Source: CAD feature listing. Evaluate the final solid. Frame: model axes, mm. A direction names the side the tool comes from. Give positions to 0.01 mm unless a question says otherwise; leave off trailing zeros. Order: outer loops, then holes, each group sorted by start corner. A loop starts at its lowest first (then second) coordinate and runs counter-clockwise, first axis right, second up.
1) Draft query along X for faces 1 (the face through (-33.44, 75.56, -0.99)), 2 (the face through (-60, 11, -1)), 3 (the face through (-91.38, 62.7, -0.99)), 4 (the face through (-33, 44, -2)). Return one class per face: released by +X, released by -X, zero draft, split by the parting line, or undercut.
2) Section C-C, the plane x = -45.5. Return loops of the section in (y, z).
3) Section B-B, the plane y = 78.5. Return loops of the section in (x, z).
4) Material intervals for line 1 (X direction, y = 45, z = -1); line 2 (Y direction, x = 27.5, z = 4.5); line 3 (Z direction, x = -79.5, y = 46.5), sorted ascending.
5) Access query for faces 5 (the face through (-33, 44, 0)), 6 (the face through (-60.1, 71.67, -0.99)), 7 (the face through (60, 11, -1)). Directions: +Z, -Z, +X, -X, +Y, -Y. A direction counts if a zero-diameter tool reaches every point of the face in a straight line with its end or side. Return the directions, or none.
6) Section A-A, the plane x = -81.5. Return loops of the section in (y, z), plus the area to 3 significant figures.
7) Section D-D, the plane z = 3. Return loops of the section in (x, y), plus the area to 3 significant figures.
8) First-contact query: P1, Ø5, axis at x = -102, z = -0.5, coming from the +Y side; P2, Ø2, axis at y = 31, z = -0.5, coming from the -X side; P3, Ø2, axis at y = 16.5, z = 0.5, coming from the -X side; P4, Ø1, axis at y = 62, z = 2, coming from the +X side. Flat tips, straight axial feed; report the tip coordinate or a pass-through.
Autodesk Inventor part; units mm, degrees
ref_plane "YZ Plane" through (0, 0, 0) normal (1, 0, 0) x (0, 1, 0)
ref_plane "XZ Plane" through (0, 0, 0) normal (0, 1, 0) x (-1, 0, 0)
ref_plane "XY Plane" through (0, 0, 0) normal (0, 0, 1) x (1, 0, 0)
sketch "草圖1" plane through (0, 0, 0) normal (0, 0, 1) x (1, 0, 0)
  line L0 (0, 0) -> (-40.5681, 0) construction
  line L1 (0, 0) -> (0, 45.2738) construction
  line L2 (-60, 18.7) -> (-21.9145, 18.7) construction
  line L3 (60, 18.1203) -> (60, 3.5)
  line L4 (56.5, 0) -> (-56.5, 0)
  line L5 (-60, 3.5) -> (-60, 18.7)
  line L6 (-87.6368, 8.7) -> (76.2221, 8.7)
  arc A0 (-60, 3.5) -> (-56.5, 0) centre (-56.5, 3.5) ccw
  arc A1 (56.5, 0) -> (60, 3.5) centre (56.5, 3.5) ccw
  arc A2 (-25, 17.157) -> (25, 17.157) centre (0, 60.4582) ccw
  line L7 (-27.5, 18.7) -> (27.5, 18.7) construction
  line L8 (16.8799, 18.7) -> (60, 18.7) construction
  line L9 (-60, 18.7) -> (-60, 20.4369)
  line L10 (-70.8518, 38.2221) -> (-119.0875, 63.0331)
  line L11 (-101.4762, 99.2795) -> (36.5219, 51.1695)
  arc A3 (-107.8929, 99.3362) -> (-124.1865, 69.3896) centre (-100.1179, 75.7) ccw
  line L12 (-104.2307, 100.2398) -> (-122.4731, 64.7746) construction
  line L13 (-92.566, 80.8091) -> (-108.8509, 80.8091)
  arc A4 (-89.2737, 80.2516) -> (-92.566, 80.8091) centre (-92.566, 70.8091) ccw
  line L14 (-32.7123, 60.5304) -> (-89.2737, 80.2516)
  arc A5 (-108.8509, 80.8091) -> (-110.452, 74.1968) centre (-108.8509, 77.3091) ccw
  line L15 (-110.452, 74.1968) -> (-70.3705, 53.5781)
  arc A6 (-70.3705, 53.5781) -> (-58.9345, 50.8091) centre (-58.9345, 75.8091) ccw
  line L16 (-58.9345, 50.8091) -> (-34.3585, 50.8091)
  arc A7 (-34.3585, 50.8091) -> (-32.7123, 60.5304) centre (-34.3585, 55.8091) ccw
  arc A8 (-88.7798, 81.668) -> (-92.566, 82.3091) centre (-92.566, 70.8091) ccw
  line L17 (-92.566, 82.3091) -> (-108.8509, 82.3091)
  arc A9 (-108.8509, 82.3091) -> (-111.1381, 72.8629) centre (-108.8509, 77.3091) ccw
  line L18 (-111.1381, 72.8629) -> (-71.0567, 52.2443)
  arc A10 (-71.0567, 52.2443) -> (-58.9345, 49.3091) centre (-58.9345, 75.8091) ccw
  line L19 (-58.9345, 49.3091) -> (-34.3585, 49.3091)
  arc A11 (-34.3585, 49.3091) -> (-32.2185, 61.9468) centre (-34.3585, 55.8091) ccw
  line L20 (-32.2185, 61.9468) -> (-88.7798, 81.668)
  arc A12 (-101.4762, 99.2795) -> (-107.8929, 99.3362) centre (-104.7682, 89.8369) ccw
  arc A13 (-124.1865, 69.3896) -> (-119.0875, 63.0331) centre (-114.5134, 71.9257) ccw
  arc A14 (25, 42.0013) -> (-25, 42.0013) centre (0, -1.3) ccw
  line L21 (-27.5, 37.6711) -> (-27.5, 21.4871)
  line L22 (27.5, 37.6711) -> (27.5, 21.4871)
  arc A15 (27.5, 37.6711) -> (25, 42.0013) centre (22.5, 37.6711) ccw
  arc A16 (25, 17.157) -> (27.5, 21.4871) centre (22.5, 21.4871) ccw
  arc A17 (-27.5, 21.4871) -> (-25, 17.157) centre (-22.5, 21.4871) ccw
  arc A18 (-25, 42.0013) -> (-27.5, 37.6711) centre (-22.5, 37.6711) ccw
  arc A19 (-60, 20.4369) -> (-70.8518, 38.2221) centre (-80, 20.4369) ccw
  arc A20 (60, 18.1203) -> (36.5219, 51.1695) centre (25, 18.1203) ccw
  point P0 (0, 0)
  point P1 (60, 42.9843)
  point P2 (-60, 40.3647)
  point P3 (-60, 32.6402)
  point P4 (27.5, 40.4582)
  point P5 (-27.5, 40.4582)
  point P6 (0, 18.7)
  dimension "d0" = 120
  dimension "d1" = 3.5
  dimension "d2" = 8.7
  dimension "d3" = 10
  dimension "d9" = 1.7582
  dimension "d12" = 117.22
  dimension "d14" = 8
  dimension "d16" = 24.8821
  dimension "d19" = 1.5
  dimension "d20" = 65
  dimension "d21" = 10
  dimension "d22" = 10
  dimension "d23" = 50
  dimension "d24" = 30
  dimension "d25" = 5
  dimension "d26" = 55
  dimension "d27" = 57
  dimension "d28" = 20
  dimension "d29" = 35
  dimension "d30" = 81.1369
extrude "擠出1" add sketch "草圖1" against normal blind 2 contours L3 L6 L5 L9 A19 L10 A13 A3 A12 L11 A20 | L3 A1 L4 A0 L5 L6
bend part "折彎零件1" radius 0.4 angle 85 line through (-87.6368, 8.7, 0) along (1, 0, 0) centre toward (0, 0, 1) moving side (0, -1, 0) both sides no
equation "\"折彎半徑\" = 厚度"
equation "\"折彎離隙寬度\" = 厚度"
equation "\"折彎離隙深度\" = 0.5 * 厚度"
equation "\"轉角離隙大小\" = 4 * 厚度"
equation "\"最小剩餘\" = 2 * 厚度"
equation "\"轉移半徑\" = 折彎半徑"
equation "\"Jacobi半徑大小\" = 折彎半徑"
equation "\"間隙大小\" = 厚度"
properties part number "0 零件" material "不鏽鋼"
From the geometry:
1. face 1: released by +X
1. face 2: released by -X
1. face 3: undercut
1. face 4: zero draft
2. outline: (5.6, 8.27) - (6.31, 0.19) arc R2.4 ccw to (8.7, -2) - (49.31, -2) - (49.31, 0) - (8.7, 0) arc R0.4 cw to (8.3, 0.37) - (7.59, 8.44) - close; (66.58, -2) - (79.76, -2) - (79.76, 0) - (66.58, 0) - close
3. outline: (-124.84, -2) - (-113.71, -2) - (-113.71, 0) - (-124.84, 0) - close; (-79.69, -2) - (-41.87, -2) - (-41.87, 0) - (-79.69, 0) - close
4. line 1: x = -84.03 to -18.88, 18.88 to 47.42
4. line 2: y = 5.93 to 7.94
4. line 3: z = -2 to 0
5. face 5: +Z, +X, -X, +Y
5. face 6: +Z, -Z
5. face 7: +Z, -Z, +X, +Y, -Y
6. outline: (43.7, -2) - (57.62, -2) - (57.62, 0) - (43.7, 0) - close; (79.13, -2) - (92.32, -2) - (92.32, 0) - (79.13, 0) - close
6. area: 54.2 mm2
7. outline: (-60, 6.06) - (60, 6.06) - (60, 8.07) - (-60, 8.07) - close
7. area: 241 mm2
8. P1: stops at y = 99.83
8. P2: stops at x = -63.68
8. P3: stops at x = -60
8. P4: passes through
